Autodesk Inventor part; units mm, degrees
ref_plane "YZ Plane" through (0, 0, 0) normal (1, 0, 0) x (0, 1, 0)
ref_plane "XZ Plane" through (0, 0, 0) normal (0, 1, 0) x (-1, 0, 0)
ref_plane "XY Plane" through (0, 0, 0) normal (0, 0, 1) x (1, 0, 0)
sketch "Эскиз2" plane through (0, 0, 0) normal (0, 0, 1) x (1, 0, 0)
  line L0 (70, 80) -> (0, 80)
  line L1 (-5, 75) -> (-5, 5)
  line L2 (75, 5) -> (75, 75)
  line L3 (0, 0) -> (70, 0)
  line L4 (70, 73.5411) -> (70, 6.4589)
  line L5 (0, 73.5411) -> (70, 73.5411)
  line L6 (0, 6.4589) -> (0, 73.5411)
  line L7 (70, 6.4589) -> (0, 6.4589)
  arc A0 (8.6686, 75.4679) -> (8.8027, 75.602) centre (7.5, 76.7706) ccw
  circle A1 centre (7.5, 76.7706) radius 1.1
  circle A2 centre (62.5, 76.7706) radius 1.1
  circle A3 centre (62.5, 3.2294) radius 1.1
  circle A4 centre (7.5, 3.2294) radius 1.1
  line L8 (-5, 75) -> (-5, 80)
  line L9 (-5, 80) -> (0, 80)
  line L10 (70, 80) -> (75, 80)
  line L11 (75, 80) -> (75, 75)
  line L12 (75, 5) -> (75, 0)
  line L13 (75, 0) -> (70, 0)
  line L14 (0, 0) -> (-5, 0)
  line L15 (-5, 5) -> (-5, 0)
  circle A5 centre (59.4102, 38.9619) radius 3.25
  circle A6 centre (59.31, 28.4306) radius 3.25
  dimension "d8" = 2.2
  dimension "d9" = 2.2
  dimension "d10" = 2.2
  dimension "d11" = 2.2
  dimension "d12" = 6.5
  dimension "d13" = 6.5
extrude "Выдавливание2" add sketch "Эскиз2" along normal blind 2 contours L10 L11 L2 L12 L13 L3 L14 L15 L1 L8 L9 L0 | L4 L7 L6 L5
fillet "Сопряжение2" radius 5 4 edges at (-5, 0, 1) (75, 0, 1) (75, 80, 1) (-5, 80, 1)
chamfer "Фаска1" distance 1.2 angle 45 4 edges at (6.4, 76.7706, 2) (61.4, 76.7706, 2) (61.4, 3.2294, 2) (6.4, 3.2294, 2)
properties part number "Case_Cover"
The listing builds one solid part. Answer for the finished solid, in the listing's coordinates (mm). Coordinates: 2 decimals unless noted, no trailing zeros. Write each loop counter-clockwise with the first axis right and the second up, starting at its lowest first coordinate (ties: lowest second). Pieces come first, ordered by that corner, then holes. Notation, with made-up numbers: (15, 28.25) - (21, 28.25) arc R12 ccw to (21, 37.25) - close; hole circle Ø10 at (54, 12.25). An arc over 180 degrees is marked (long way). Return JSON: item names as keys, results as strings. Group by question number.
Q1. Find the intervals of material crossed by line 1 along Y through (x, z) = (7.5, 0.55); line 2 along Y through (x, z) = (59.31, 0.4), in increasing order. Write a range as [from, to].
Q2. For a pull along Y with two mould halves and no side action, classify faces 1 (the cylindrical face through (62.41, 27.45, 0.99)), 2 (the flat face through (35, 0, 1)), 3 (the flat face through (34, 41, 2)) as +Y half, -Y half, draft (parallel to the pull), parting line (faces both ways), or undercut.
Q3. Flat-ended cylindrical pins translate along their axes: pin 1 Ø5 at (x, y) = (59.31, 28.43) entering from +Z; pin 2 Ø2.5 at (x, y) = (7.5, 3.23) entering from +Z; pin 3 Ø3 at (x, y) = (7.5, 76.77) entering from +Z; pin 4 Ø3.5 at (x, y) = (62.5, 76.77) entering from +Z. Find the tip coordinate at first contact, or state that the pin passes through.
Q4. The part is cut by section A-A on z = 1.25. Write down the section's boundary in (x, y).
Evaluation:
{
 "1": {"line 1": "y = [0, 2.13], [4.33, 75.67], [77.87, 80]", "line 2": "y = [0, 25.18], [31.68, 35.71], [42.21, 80]"},
 "2": {"face 1": "undercut", "face 2": "-Y half", "face 3": "draft"},
 "3": {"pin 1": "passes through", "pin 2": "stops at z = 0.95", "pin 3": "stops at z = 1.2", "pin 4": "stops at z = 1.45"},
 "4": {"outline": "(-5, 5) arc R5 ccw to (0, 0) - (70, 0) arc R5 ccw to (75, 5) - (75, 75) arc R5 ccw to (70, 80) - (0, 80) arc R5 ccw to (-5, 75) - close; hole circle Ø3.1 at (7.5, 3.23); hole circle Ø3.1 at (7.5, 76.77); hole circle Ø6.5 at (59.31, 28.43); hole circle Ø6.5 at (59.41, 38.96); hole circle Ø3.1 at (62.5, 3.23); hole circle Ø3.1 at (62.5, 76.77)"}
}
